Could you check a few things on this model? Use its own coordinates, in mm. Round coordinates to 2 decimals unless told otherwise and drop trailing zeros. Write each loop counter-clockwise with the first axis right and the second up, starting at its lowest first coordinate (ties: lowest second). Pieces come first, ordered by that corner, then holes. Notation, with made-up numbers: (71, -4.75) -> (84, -4.75) arc R16 ccw to (84, 17.25) -> close; hole circle Ø9 at (29.5, 83.5). An arc over 180 degrees is marked (long way). Answer in a Markdown table with one row per item.
from build123d import *

# Parameters (mm, degrees)
SKETCH3_R           = 22.5
SKETCH3_R_2         = 19
BOSS_EXTRUDE1_DEPTH = 4.7
FILLET1_R           = 2
FILLET2_R           = 2


with BuildPart() as part:
    # Sketch3 → Boss-Extrude1 (new body)
    with BuildSketch(Plane(origin=(0, 0, 0), x_dir=(1, 0, 0), z_dir=(0, 1, 0))):
        with Locations(Location((0, 0, 0), (0, 0, 270))):
            Circle(SKETCH3_R)
        with Locations(Location((0, 0, 0), (0, 0, 270))):
            Circle(SKETCH3_R_2, mode=Mode.SUBTRACT)
    extrude(amount=BOSS_EXTRUDE1_DEPTH)

    # Fillet1
    fillet1_edges = [part.edges().sort_by_distance(p)[0] for p in [
        (0, 0, -19),
        (0, 4.7, -19),
    ]]
    fillet(fillet1_edges, radius=FILLET1_R)

    # Fillet2
    # the kernel refuses this fillet: 2 mm, written as the material it takes off along each edge
    with BuildSketch(Plane(origin=(0, 0, 0), x_dir=(0, 0, 1), z_dir=(-1, 0, 0))) as fillet2_piece_1:
        with BuildLine():
            CenterArc((20.5, 1.936491673), FILLET2_R, 284.477512186, 75.522487814)
            Line((22.5, 1.936491673), (22.54, 1.936491673))
            Line((22.54, 1.936491673), (22.54, 0))
            Line((22.54, 0), (22.5, -0.04))
            ThreePointArc((22.5, -0.04), (21.75, -0.04), (21.01, -0.038729833))
            Line((21.01, -0.038729833), (21, 0))
        make_face()
    revolve(axis=Axis((0, 0, 0), (0, 1, 0)), mode=Mode.SUBTRACT)
    with BuildSketch(Plane(origin=(0, 4.7, 0), x_dir=(0, 0, 1), z_dir=(-1, 0, 0))) as fillet2_piece_2:
        with BuildLine():
            CenterArc((20.5, -1.936491673), FILLET2_R, 0, 75.522487814)
            Line((22.5, -1.936491673), (22.54, -1.936491673))
            Line((22.54, -1.936491673), (22.54, 0))
            Line((22.54, 0), (22.5, 0.04))
            ThreePointArc((22.5, 0.04), (21.75, 0.04), (21.01, 0.038729833))
            Line((21.01, 0.038729833), (21, 0))
        make_face()
    revolve(axis=Axis((0, 4.7, 0), (0, 1, 0)), mode=Mode.SUBTRACT)


solid = part.part
1) Please list where these lines run through material, in increasing order: line 1 (X direction, y = 2.5, z = 0); line 2 (Z direction, x = -17, y = 3.85); line 3 (Z direction, x = 8.5, y = 3.4).
Findings:
| item | result |
|---|---|
| line 1 | x = -22.5 to -19, 19 to 22.5 |
| line 2 | z = -14.24 to -9.27, 9.27 to 14.24 |
| line 3 | z = -20.72 to -17.13, 17.13 to 20.72 |
2) Imagine slicing it at C-C, the plane y = 1.2. Please give me the cut outline in (x, z), plus the area to 3 significant figures.
Findings:
| item | result |
|---|---|
| outline | circle Ø44.72 at (0, 0); hole circle Ø38.33 at (0, 0) |
| area | 416 mm^2 |
3) Imagine slicing it at B-B, the plane y = 3.55. Please give me the cut outline in (x, z), plus the area to 3 significant figures.
Findings:
| item | result |
|---|---|
| outline | circle Ø44.68 at (0, 0); hole circle Ø38.38 at (0, 0) |
| area | 411 mm^2 |
4) Imagine slicing it at A-A, the plane z = 0. Please give me the cut outline in (x, y).
Findings:
| item | result |
|---|---|
| outline | (-22.5, 1.94) arc R2 ccw to (-21, 0) arc R2 ccw to (-19, 2) -> (-19, 2.7) arc R2 ccw to (-21, 4.7) arc R2 ccw to (-22.5, 2.76) -> close; (19, 2) arc R2 ccw to (21, 0) arc R2 ccw to (22.5, 1.94) -> (22.5, 2.76) arc R2 ccw to (21, 4.7) arc R2 ccw to (19, 2.7) -> close |
5) Thinking about a two-plate mould opening in Z: for faces 1 (the face through (-8.618, 2.344, 20.784)), 2 (the face through (-11.56, 2.35, -15.08)), which applies, +Z half, -Z half, draft (parallel to the pull), parting line (faces both ways), or undercut?
Findings:
| item | result |
|---|---|
| face 1 | parting line |
| face 2 | undercut |
